Input: part model. Units: mm. Frame: model coordinates. Face numbers are marked on the shaded views. A direction names the side the tool comes from. Round coordinates to 2 decimals unless told otherwise and drop trailing zeros. Order: outer loops, then holes, each group sorted by start corner. A loop starts at its lowest first (then second) coordinate and runs counter-clockwise, first axis right, second up. Notation, with made-up numbers: (-7.5, -27) -> (31.5, -27) arc R6 cw to (31.5, -19) -> close; hole circle Ø7 at (23.25, 72.25). An arc over 180 degrees is marked (long way). Use a Markdown table: item, result.
from build123d import *

# Parameters (mm, degrees)
SKETCH_R      = 4
PAD_DEPTH     = 2
SKETCH002_R   = 7
SKETCH002_R_2 = 4
PAD001_DEPTH  = 10
SKETCH003_R   = 6
SKETCH003_R_2 = 4
PAD002_DEPTH  = 2
SKETCH004_R   = 4
SKETCH004_R_2 = 3
SKETCH004_W   = 6
SKETCH004_H   = 3
PAD003_DEPTH  = 2
POCKET_DEPTH  = 5


with BuildPart() as part:
    # Sketch → Pad (new body)
    with BuildSketch(Plane.XY):
        with BuildLine():
            ThreePointArc((-33, 30), (-34.414214, 29.414214), (-35, 28))
            Line((-35, -23), (-35, 28))
            ThreePointArc((-35, -23), (-34.414214, -24.414214), (-33, -25))
            Line((23, -25), (-33, -25))
            ThreePointArc((23, -25), (24.414214, -24.414214), (25, -23))
            Line((25, 28), (25, -23))
            ThreePointArc((25, 28), (24.414214, 29.414214), (23, 30))
            Line((-33, 30), (23, 30))
        make_face()
        Circle(SKETCH_R, mode=Mode.SUBTRACT)
    extrude(amount=PAD_DEPTH)

    # Sketch002 (on Face10 of Pad) → Pad001 (join)
    with BuildSketch(Plane(origin=(0, 0, 0), x_dir=(1, 0, 0), z_dir=(0, 0, -1))):
        Circle(SKETCH002_R)
        Circle(SKETCH002_R_2, mode=Mode.SUBTRACT)
    extrude(amount=PAD001_DEPTH)

    # Sketch003 (on Face12 of Pad001) → Pad002 (join)
    with BuildSketch(Plane(origin=(0, 0, -10), x_dir=(1, 0, 0), z_dir=(0, 0, -1))):
        Circle(SKETCH003_R)
        Circle(SKETCH003_R_2, mode=Mode.SUBTRACT)
    extrude(amount=PAD002_DEPTH)

    # Sketch004 (on Face4 of Pad002) → Pad003 (join)
    with BuildSketch(Plane(origin=(0, 0, 0), x_dir=(1, 0, 0), z_dir=(0, 0, -1))):
        with Locations((-23, -24)):
            Circle(SKETCH004_R)
        with Locations((20.5, -20)):
            Circle(SKETCH004_R_2)
        with Locations((17.5, 23.5)):
            Rectangle(SKETCH004_W, SKETCH004_H)
        with Locations((-24.5, 23.5)):
            Rectangle(SKETCH004_W, SKETCH004_H)
    extrude(amount=PAD003_DEPTH)

    # Sketch005 (on Face4 of Pad003) → Pocket (cut)
    with BuildSketch(Plane(origin=(0, 0, 0), x_dir=(1, 0, 0), z_dir=(0, 0, -1))):
        with BuildLine():
            ThreePointArc((24, 20), (22.75, 18.75), (24, 17.5))
            Line((24, 17.5), (25, 17.5))
            Line((25, 20), (25, 17.5))
            Line((24, 20), (25, 20))
        make_face()
    extrude(amount=-POCKET_DEPTH, mode=Mode.SUBTRACT)


solid = part.part
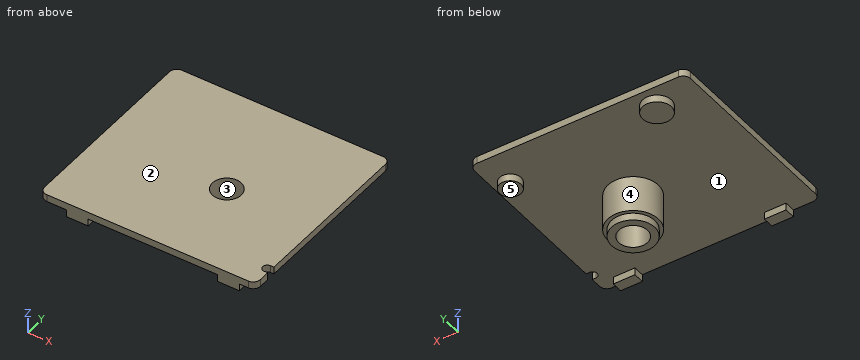
1) Cut plane B-B on y = 0. Return loops of the section in (x, z).
Results found:
| item | result |
|---|---|
| outline | (-35, 0) -> (-7, 0) -> (-7, -10) -> (-6, -10) -> (-6, -12) -> (-4, -12) -> (-4, 2) -> (-35, 2) -> close; (4, -12) -> (6, -12) -> (6, -10) -> (7, -10) -> (7, 0) -> (25, 0) -> (25, 2) -> (4, 2) -> close |
2) Cut plane A-A on x = 0. Return loops of the section in (y, z).
Results found:
| item | result |
|---|---|
| outline | (-25, 0) -> (-7, 0) -> (-7, -10) -> (-6, -10) -> (-6, -12) -> (-4, -12) -> (-4, 2) -> (-25, 2) -> close; (4, -12) -> (6, -12) -> (6, -10) -> (7, -10) -> (7, 0) -> (30, 0) -> (30, 2) -> (4, 2) -> close |
3) Cut plane D-D on y = -18.75. Return loops of the section in (x, z), and give its area (4 significant figures).
Results found:
| item | result |
|---|---|
| outline | (-35, 0) -> (22.75, 0) -> (22.75, 2) -> (-35, 2) -> close |
| area | 115.5 mm² |
4) Cut plane C-C on x = -23. Return loops of the section in (y, z).
Results found:
| item | result |
|---|---|
| outline | (-25, -2) -> (-22, -2) -> (-22, 0) -> (20, 0) -> (20, -2) -> (28, -2) -> (28, 0) -> (30, 0) -> (30, 2) -> (-25, 2) -> close |
5) Line query: L1, parallel to X at y = 0, z = -3.25; L2, parallel to Z at x = -11, y = -0.5. Output: solid intervals per line, ascending. Write a range as [from, to].
Results found:
| item | result |
|---|---|
| L1 | x = [-7, -4], [4, 7] |
| L2 | z = [0, 2] |
6) Pin query (flat end, axial travel): pin 1 Ø1 at (x, z) = (-14.5, -2) entering from +Y; pin 2 Ø1.1 at (x, z) = (24.5, 0.5) entering from -Y; pin 3 Ø2.5 at (x, y) = (-26, -24) entering from -Z; pin 4 Ø6 at (y, z) = (3, -8.5) entering from -X. Return the tip coordinate at first contact, or that it passes through.
Results found:
| item | result |
|---|---|
| pin 1 | passes through |
| pin 2 | stops at y = -24.76 |
| pin 3 | stops at z = -2 |
| pin 4 | stops at x = -7 |
7) Set-up query: the marked faces 1 and 2. Return all of +Z, -Z, +X, -X, +Y, -Y with unobstructed straight access to the full face (end or side cutting, diameter ignored); none if empty.
Results found:
| item | result |
|---|---|
| face 1 | -Z |
| face 2 | +Z, +X, -X, +Y, -Y |
8) Pull-direction query (Y, two-part tool) for the marked faces 3, 4 and 5; classes: +Y half, -Y half, draft (parallel to the pull), parting line (faces both ways), or undercut.
Results found:
| item | result |
|---|---|
| face 3 | undercut |
| face 4 | parting line |
| face 5 | draft |
